from build123d import *

# Parameters (mm, degrees)
SKETCH1_R           = 1.5875
BOSS_EXTRUDE1_DEPTH = 6.35


with BuildPart() as part:
    # Sketch1 → Boss-Extrude1 (new body)
    with BuildSketch(Plane(origin=(0, 0, 0), x_dir=(1, 0, 0), z_dir=(0, 1, 0))):
        Polygon((-75.214775388, -28.322289224), (153.385224612, -28.322289224), (153.385224612, -41.022289224), (159.735224612, -41.022289224), (159.735224612, -66.422289224), (159.735224612, -91.822289224), (153.385224612, -91.822289224), (153.385224612, -104.522289224), (-75.214775388, -104.522289224), (-75.214775388, -79.122289224), (-81.564775388, -79.122289224), (-81.564775388, -53.722289224), (-75.214775388, -53.722289224), align=None)
        with Locations(Location((156.560224612, -53.722289224, 0), (0, 0, 270))):
            Circle(SKETCH1_R, mode=Mode.SUBTRACT)
        with Locations(Location((156.560224612, -79.122289224, 0), (0, 0, 270))):
            Circle(SKETCH1_R, mode=Mode.SUBTRACT)
    extrude(amount=BOSS_EXTRUDE1_DEPTH)


solid = part.part
Geometry check sheet. Reference: the model listing, model coordinates, mm. A direction names the side the tool comes from. Round coordinates to 2 decimals unless told otherwise and drop trailing zeros. Loops run counter-clockwise (first coordinate to the right, second up) from the corner with the lowest first, then second, coordinate; pieces in that order, holes last.
Item 1: Cross-section at C-C on z = 85. Record the boundary of the cut face in (x, y).
Item 2: Thickness scan on line 1 (X direction, y = 2, z = 35); line 2 (X direction, y = 3.5, z = 79.5); line 3 (X direction, y = 1.25, z = 84.5). Record the ranges inside material, lowest first.
Item 3: Cross-section at A-A on y = 5. Record the boundary of the cut face in (x, z) (1 decimal).
Item 4: Access from +Z, -Z, +X, -X, +Y, -Y to the whole of each face (thin tool, end or side, straight path). Record for faces 1 (the flat face through (-75.215, 3, 41)), 2 (the flat face through (157, 3, 91.822)), 3 (the flat face through (-78, 3, 79.122)), 4 (the flat face through (153.385, 3, 35)).
Item 5: Cross-section at B-B on z = 97.5. Record the boundary of the cut face in (x, y), then the cut area to 3 significant figures.
Item 6: Gauge pin test, flat ends, axial feed: pin 1 (3 mm diameter, centred on y = 3.5, z = 46, fed in from -X); pin 2 (1 mm diameter, centred on y = 4, z = 39, fed in from +X); pin 3 (1.9 mm diameter, centred on x = -79.5, y = 4.5, fed in from +Z); pin 4 (5 mm diameter, centred on x = 156.56, z = 79.12, fed in from +Y). Record the tip position at first contact, or that the pin passes through.
Answer sheet:
1. outline: (-75.21, 0) - (159.74, 0) - (159.74, 6.35) - (-75.21, 6.35) - close
2. line 1: x = -75.21 to 153.39
2. line 2: x = -75.21 to 155.02, 158.1 to 159.74
2. line 3: x = -75.21 to 159.74
3. outline: (-81.6, 53.7) - (-75.2, 53.7) - (-75.2, 28.3) - (153.4, 28.3) - (153.4, 41) - (159.7, 41) - (159.7, 91.8) - (153.4, 91.8) - (153.4, 104.5) - (-75.2, 104.5) - (-75.2, 79.1) - (-81.6, 79.1) - close; hole circle Ø3.2 at (156.6, 53.7); hole circle Ø3.2 at (156.6, 79.1)
4. face 1: -Z, -X, +Y, -Y
4. face 2: +Z, +X, +Y, -Y
4. face 3: +Z, -X, +Y, -Y
4. face 4: -Z, +X, +Y, -Y
5. outline: (-75.21, 0) - (153.39, 0) - (153.39, 6.35) - (-75.21, 6.35) - close
5. area: 1,450 mm2
6. pin 1: stops at x = -75.21
6. pin 2: stops at x = 153.39
6. pin 3: stops at z = 79.12
6. pin 4: stops at y = 6.35
